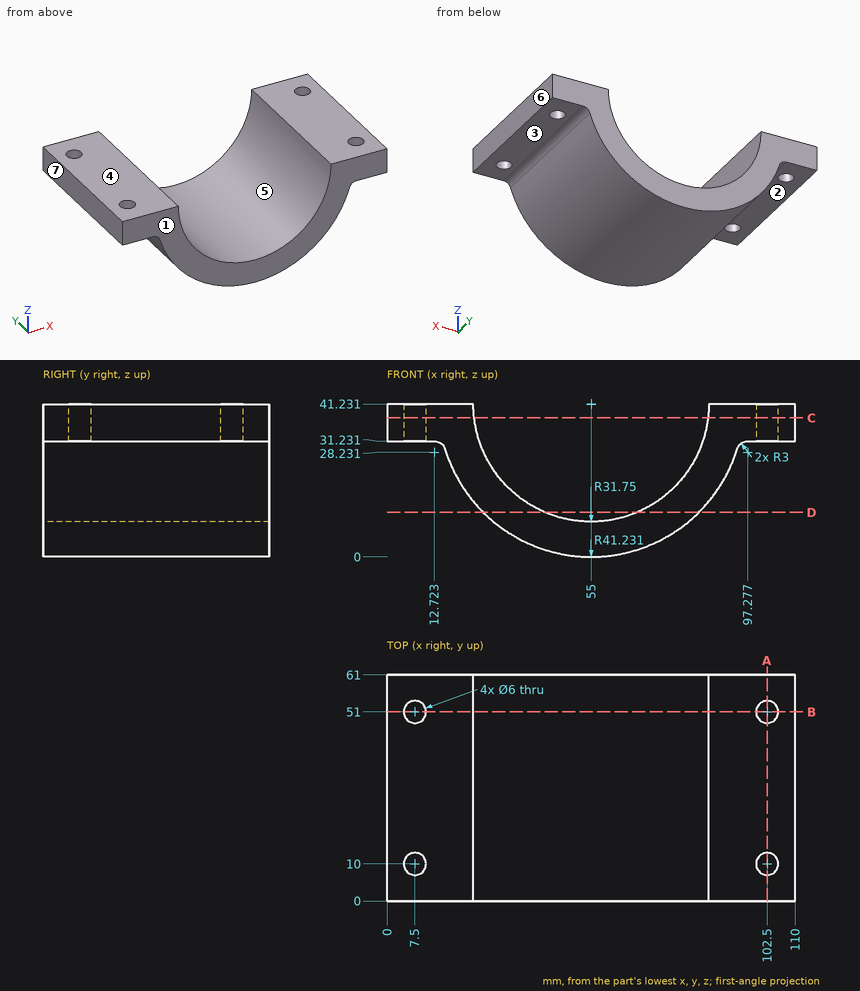
Part print with two shaded views. Sizes in mm from the minimum x, y, z corner. A direction names the side the tool comes from. Round coordinates to 2 decimals unless told otherwise and drop trailing zeros. Loops run counter-clockwise (first coordinate to the right, second up) from the corner with the lowest first, then second, coordinate; pieces in that order, holes last. Notation, with made-up numbers: (28, 66.25) - (72, 66.25) arc R15 cw to (72, 92.25) - close; hole circle Ø10 at (40.5, -7.75). An arc over 180 degrees is marked (long way). Answer as a JSON object with one key per item and string values.
Item 1: Pin check, flat tips, straight feed: pin 1 (6.5 mm diameter, centred on x = 4, y = 45, fed in from -Z); pin 2 (5 mm diameter, centred on y = 23, z = 15, fed in from +X); pin 3 (5 mm diameter, centred on x = 53.5, y = 46, fed in from +Z); pin 4 (7 mm diameter, centred on x = 102.5, y = 10, fed in from +Z). Stop position of each tip, or through.
Output:
{"pin 1": "z = 31.23", "pin 2": "x = 88.72", "pin 3": "z = 9.73", "pin 4": "z = 41.23"}
Item 2: Wall check: L1, parallel to Y at x = 102.5, z = 35.5; L2, parallel to X at y = 51, z = 38 (1 decimal); L3, parallel to X at y = 10, z = 34 (1 decimal). Give the ranges that are in metal, low to high.
Output:
{"L1": "0 to 7, 13 to 48, 54 to 61", "L2": "0 to 4.5, 10.5 to 23.4, 86.6 to 99.5, 105.5 to 110", "L3": "0 to 4.5, 10.5 to 24.1, 85.9 to 99.5, 105.5 to 110"}
Item 3: Band-saw the part on A-A on x = 102.5. List the corners of the cut face in (y, z).
Output:
{"outline": "(0, 31.23) - (7, 31.23) - (7, 41.23) - (0, 41.23) - close; (13, 31.23) - (48, 31.23) - (48, 41.23) - (13, 41.23) - close; (54, 31.23) - (61, 31.23) - (61, 41.23) - (54, 41.23) - close"}
Item 4: Tool access for the marked faces 1, 2 and 3: list every direction of +Z, -Z, +X, -X, +Y, -Y with a clear straight run to the whole face (end or side of a thin tool).
Output:
{"face 1": "+Z, -Z, +X, -X, -Y", "face 2": "-Z, -X, +Y, -Y", "face 3": "-Z, +X, +Y, -Y"}
Item 5: Band-saw the part on B-B on y = 51. List the corners of the cut face in (x, z).
Output:
{"outline": "(0, 31.23) - (4.5, 31.23) - (4.5, 41.23) - (0, 41.23) - close; (10.5, 31.23) - (12.72, 31.23) arc R3 cw to (15.59, 29.11) arc R41.23 ccw to (94.41, 29.11) arc R3 cw to (97.28, 31.23) - (99.5, 31.23) - (99.5, 41.23) - (86.75, 41.23) arc R31.75 cw to (23.25, 41.23) - (10.5, 41.23) - close; (105.5, 31.23) - (110, 31.23) - (110, 41.23) - (105.5, 41.23) - close"}
Item 6: Band-saw the part on D-D on z = 12. List the corners of the cut face in (x, y).
Output:
{"outline": "(25.92, 0) - (42.61, 0) - (42.61, 61) - (25.92, 61) - close; (67.39, 0) - (84.08, 0) - (84.08, 61) - (67.39, 61) - close"}
Item 7: Pull direction X, two halves, no side cores. Call the marked faces 4, 5, 6 and 7: pulls with the +X half, pulls with the -X half, needs draft (parallel to the pull), parting line crosses it, or undercut.
Output:
{"face 4": "needs draft", "face 5": "undercut", "face 6": "pulls with the +X half", "face 7": "pulls with the -X half"}
Item 8: Band-saw the part on C-C on z = 37.5. List the corners of the cut face in (x, y), plus the area to 3 significant figures.
Output:
{"outline": "(0, 0) - (23.47, 0) - (23.47, 61) - (0, 61) - close; (86.53, 0) - (110, 0) - (110, 61) - (86.53, 61) - close; hole circle Ø6 at (7.5, 10); hole circle Ø6 at (7.5, 51); hole circle Ø6 at (102.5, 10); hole circle Ø6 at (102.5, 51)", "area": "2,750 mm2"}
